Geometry: see drawing. Coordinates: mm, zero at the bounding-box minimum. A direction names the side the tool comes from. Give positions to 0.01 mm unless a question says otherwise; leave off trailing zeros. Write each loop counter-clockwise with the first axis right and the second up, starting at its lowest first coordinate (ties: lowest second). Pieces come first, ordered by that corner, then holes. Notation, with made-up numbers: M 52,61 L 64,61 A31 cw 64,100 Z; hole C 46.25,5.25 d2. An arc over 180 degrees is marked long. Use a Markdown table: item, result. Add a question column.
(1) Pin query (flat end, axial travel): pin 1 Ø1 at (y, z) = (21.5, 41.5) entering from -X; pin 2 Ø4 at (x, z) = (35, 19.5) entering from -Y; pin 3 Ø2 at (x, y) = (33.5, 16.5) entering from +Z; pin 4 Ø3 at (x, y) = (40.5, 22) entering from -Z. Return the tip coordinate at first contact, or that it passes through.
(2) Cut plane A-A (z = 17). Output: boundary loops of the cut face in (x, y).
(3) Material intervals for L1, parallel to X at y = 11, z = 34.5; L2, parallel to X at y = 21.75, z = 55; L3, parallel to Y at x = 54, z = 29.5, sorted ascending.
(4) Cut plane D-D (y = 8.5). Output: boundary loops of the cut face in (x, z).
(5) Reachability of the marked faces 1 and 2 from +Z, -Z, +X, -X, +Y, -Y: full face, straight path, thin tool, end or side. Return the list, or none.
(6) Cut plane C-C (x = 35). Output: boundary loops of the cut face in (y, z), plus the area to 3 significant figures.
(7) Cut plane B-B (y = 2). Output: boundary loops of the cut face in (x, z), plus the area to 3 significant figures.
(8) Draft query along X for the marked faces 3, 4, 5 and 6. Return one class per face: released by +X, released by -X, zero draft, split by the parting line, or undercut.
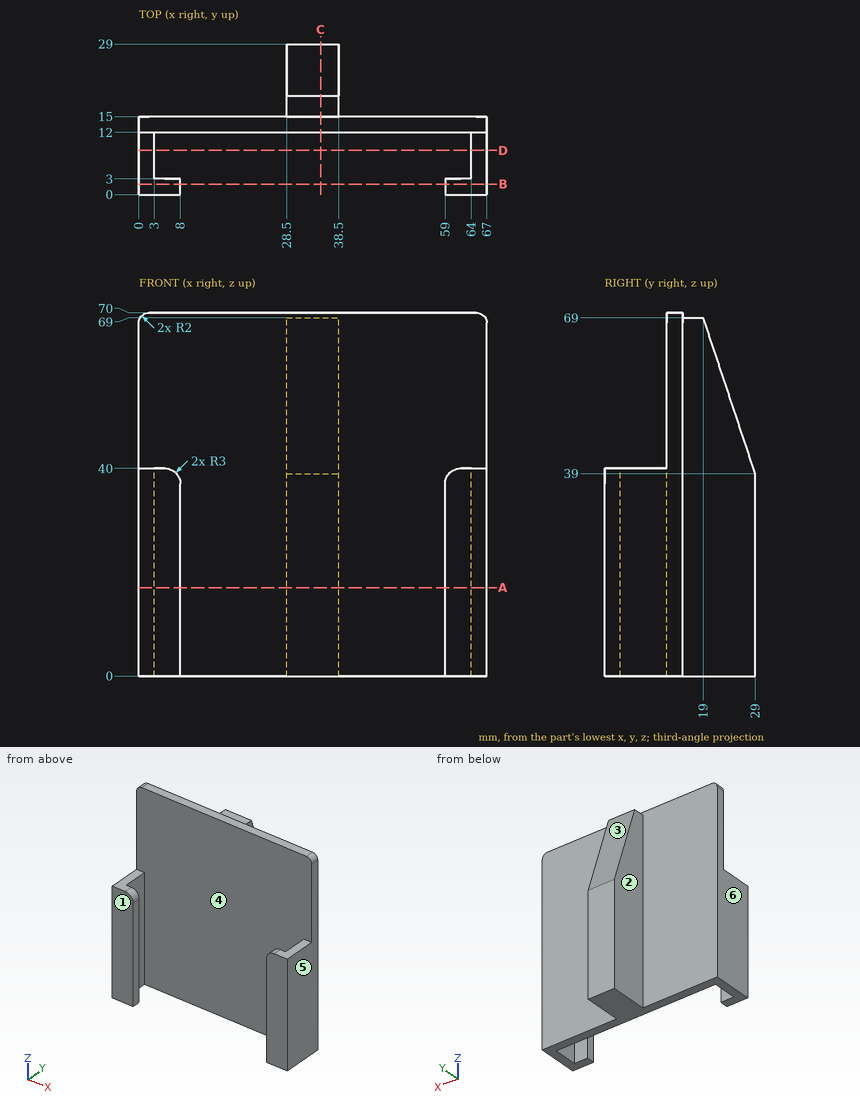
Answer list:
| question | item | result |
|---|---|---|
| 1 | pin 1 | x = 28.5 |
| 1 | pin 2 | y = 12 |
| 1 | pin 3 | z = 69 |
| 1 | pin 4 | through |
| 2 | outline | M 0,0 L 8,0 L 8,3 L 3,3 L 3,12 L 64,12 L 64,3 L 59,3 L 59,0 L 67,0 L 67,15 L 38.5,15 L 38.5,29 L 28.5,29 L 28.5,15 L 0,15 Z |
| 3 | L1 | 0 to 3, 64 to 67 |
| 3 | L2 | 28.5 to 38.5 |
| 3 | L3 | 12 to 15 |
| 4 | outline | M 0,0 L 3,0 L 3,40 L 0,40 Z; M 64,0 L 67,0 L 67,40 L 64,40 Z |
| 5 | face 1 | +Z, -Z, +X, -X, -Y |
| 5 | face 2 | +Z, -Z, -X, +Y |
| 6 | outline | M 12,0 L 29,0 L 29,39 L 19,69 L 15,69 L 15,70 L 12,70 Z |
| 6 | area | 1,030 mm² |
| 7 | outline | M 0,0 L 8,0 L 8,37 A3 ccw 5,40 L 0,40 Z; M 59,0 L 67,0 L 67,40 L 62,40 A3 ccw 59,37 Z |
| 7 | area | 636 mm² |
| 8 | face 3 | zero draft |
| 8 | face 4 | undercut |
| 8 | face 5 | released by +X |
| 8 | face 6 | released by -X |
